```python
from build123d import *

# Parameters (mm, degrees)
SKETCH1_R           = 15
BOSS_EXTRUDE1_DEPTH = 3
BOSS_EXTRUDE4_DEPTH = 3
BOSS_EXTRUDE5_DEPTH = 3
SKETCH4_R           = 1.5
CUT_EXTRUDE1_DEPTH  = 3


with BuildPart() as part:
    # Sketch1 → Boss-Extrude1 (new body)
    with BuildSketch(Plane(origin=(0, 0, 0), x_dir=(1, 0, 0), z_dir=(0, 1, 0))):
        with Locations(Location((0, 0, 0), (0, 0, 270))):
            Circle(SKETCH1_R)
    extrude(amount=BOSS_EXTRUDE1_DEPTH)

    # Sketch2 → Boss-Extrude4 (add)
    with BuildSketch(Plane(origin=(0, 3, 0), x_dir=(1, 0, 0), z_dir=(0, 1, 0))):
        Polygon((1.75, -22.853946612), (-1.75, -22.853946612), (-4, -14.456832295), (4, -14.456832295), align=None)
        Polygon((-14.848992515, -17.460607006), (-11.733580795, -9.344682002), (-5.26144484, -14.04696402), (-12.017433035, -19.517855389), align=None)
        Polygon((-22.276174588, -5.397908988), (-14.985332536, -0.663180799), (-12.513196581, -8.271632929), (-21.194615108, -8.726606795), align=None)
        Polygon((-21.194615108, 8.726606795), (-12.513196581, 8.271632929), (-14.985332536, 0.663180799), (-22.276174588, 5.397908988), align=None)
        Polygon((-12.017433035, 19.517855389), (-5.26144484, 14.04696402), (-11.733580795, 9.344682002), (-14.848992515, 17.460607006), align=None)
        Polygon((1.75, 22.853946612), (4, 14.456832295), (-4, 14.456832295), (-1.75, 22.853946612), align=None)
        Polygon((14.848992515, 17.460607006), (11.733580795, 9.344682002), (5.26144484, 14.04696402), (12.017433035, 19.517855389), align=None)
        Polygon((22.276174588, 5.397908988), (14.985332536, 0.663180799), (12.513196581, 8.271632929), (21.194615108, 8.726606795), align=None)
        Polygon((21.194615108, -8.726606795), (12.513196581, -8.271632929), (14.985332536, -0.663180799), (22.276174588, -5.397908988), align=None)
        Polygon((12.017433035, -19.517855389), (5.26144484, -14.04696402), (11.733580795, -9.344682002), (14.848992515, -17.460607006), align=None)
    extrude(amount=-BOSS_EXTRUDE4_DEPTH)

    # Sketch3 → Boss-Extrude5 (add)
    with BuildSketch(Plane(origin=(0, 3, 0), x_dir=(1, 0, 0), z_dir=(0, 1, 0))):
        Polygon((0, 0), (5.26144484, 14.04696402), (22.895002409, 38.317473852), (29.367138364, 33.615191833), (11.733580795, 9.344682002), align=None)
    extrude(amount=-BOSS_EXTRUDE5_DEPTH)

    # Sketch4 → Cut-Extrude1 (cut)
    with BuildSketch(Plane(origin=(0, 3, 0), x_dir=(1, 0, 0), z_dir=(0, 1, 0))):
        with Locations(Location((0, 0, 0), (0, 0, 270))):
            Circle(SKETCH4_R)
    extrude(amount=-CUT_EXTRUDE1_DEPTH, mode=Mode.SUBTRACT)


solid = part.part
```
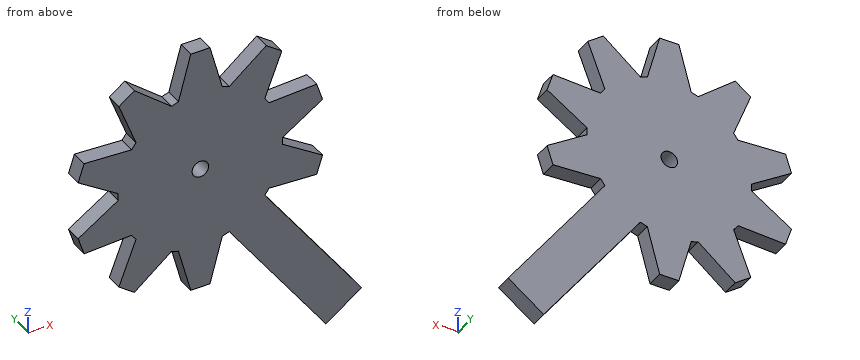
Design review of the part built by this model. Coordinates are the model's own, in mm. Round coordinates to 2 decimals unless told otherwise and drop trailing zeros. Order: outer loops, then holes, each group sorted by start corner. A loop starts at its lowest first (then second) coordinate and runs counter-clockwise, first axis right, second up. Notation, with made-up numbers: M 3,-36 L 49,-36 A19 cw 49,-9 Z; hole C 57.25,25 d5. An arc over 180 degrees is marked long. Put each result on its own line as item: value.
Q1. Consider section B-B (x = 0). State the section outline as (y, z) points.
Reported:
outline: M 0,-22.85 L 3,-22.85 L 3,-1.5 L 0,-1.5 Z; M 0,1.5 L 3,1.5 L 3,22.85 L 0,22.85 Z
Q2. Consider section C-C (x = 17.5). State the section outline as (y, z) points, and give its area (3 significant figures).
Reported:
outline: M 0,-30.89 L 3,-30.89 L 3,-17.28 L 0,-17.28 Z; M 0,-8.53 L 3,-8.53 L 3,-2.3 L 0,-2.3 Z; M 0,2.3 L 3,2.3 L 3,8.53 L 0,8.53 Z
area: 78.3 mm²
Q3. Consider section D-D (z = -12). State the section outline as (x, y) points.
Reported:
outline: M -12.75,0 L 13.66,0 L 13.66,3 L -12.75,3 Z
Q4. Insertion check: pin 1 Ø1.8 at (x, z) = (0, 0) entering from +Y; pin 2 Ø5 at (x, z) = (22.5, -10) entering from -Y. Each pin has a flat end and moves straight along its axis. Give the tip position at first contact, or say it passes through.
Reported:
pin 1: through
pin 2: y = 0
Q5. To check wall thickness, follow line 1 (X direction, y = 1.4, z = 14.5); line 2 (X direction, y = 1.05, z = 0); line 3 (X direction, y = 1.05, z = -15.5). State the ranges of each line that lie inside material, in increasing order.
Reported:
line 1: -13.71 to -5.82, -3.99 to 3.99, 5.82 to 13.71
line 2: -15 to -1.5, 1.5 to 15
line 3: -14.1 to -7.06, -3.72 to 3.72, 6.32 to 16.21
Q6. Consider section A-A (z = 0). State the section outline as (x, y) points.
Reported:
outline: M -15,0 L -1.5,0 L -1.5,3 L -15,3 Z; M 1.5,0 L 15,0 L 15,3 L 1.5,3 Z
